from build123d import *
from build123d.topology import SkipClean

# Parameters (mm, degrees)
SKETCH4_R           = 1.524
BOSS_EXTRUDE1_DEPTH = 0.9906
FILLET1_R           = 1.27


with BuildPart() as part:
    # Sketch4 → Boss-Extrude1 (new, symmetric)
    with BuildSketch(Plane.XY):
        with BuildLine():
            Line((-18.252177815, -23.016396438), (-23.016396438, -23.016396438))
            ThreePointArc((-23.016396438, -23.016396438), (-28.612162641, 10.693388458), (0, 29.3751))
            Line((0, 29.3751), (0, 35.7251))
            ThreePointArc((0, 35.7251), (-35.708437486, 1.090991438), (-2.18096518, -35.658465487))
            Line((-2.18096518, -35.658465487), (-1.793306954, -29.320309517))
            ThreePointArc((-1.793306954, -29.320309517), (-10.506673828, -27.431848371), (-18.252177815, -23.016396438))
        make_face()
        with Locations((-7.598669938, -31.650738146)):
            Circle(SKETCH4_R, mode=Mode.SUBTRACT)
    extrude(amount=BOSS_EXTRUDE1_DEPTH, both=True)

    # Fillet1
    fillet1_edges = [part.edges().sort_by_distance(p)[0] for p in [
        (-23.016396438, -23.016396438, 0),
    ]]
    fillet(fillet1_edges, radius=FILLET1_R)

    # Mirror1: part across plane


with BuildPart() as part_1:
    with SkipClean():  # the faces are left unmerged after this step: merging them gives an invalid solid
        add(part.part)
        add(part.part.mirror(Plane(origin=(0, 0, 0), x_dir=(0, 0, 1), z_dir=(1, 0, 0))))


solid = part_1.part
The model under review builds one solid part; all positions refer to its coordinate system, in mm. A direction names the side the tool comes from. Round coordinates to 2 decimals unless told otherwise and drop trailing zeros. Loops run counter-clockwise (first coordinate to the right, second up) from the corner with the lowest first, then second, coordinate; pieces in that order, holes last. Notation, with made-up numbers: M -36.5,3 L -6.5,3 A21 cw -6.5,20 Z; hole C -38,83.5 d6. An arc over 180 degrees is marked long. Answer as CSV lines item,"result". Start each with the question number.
Item 1: For faces 4 (the face through (-5.1, 29.3, 0.991)), 5 (the face through (20, -23.016, 0)), 6 (the face through (-1.99, -32.53, 0.01)), list the 3-axis set-ups (+Z, -Z, +X, -X, +Y, -Y) from which the entire face can be reached by the end or side of a thin tool; tool diameter is ignored.
Item 2: Mouldability with a two-part tool opening along Y and no side actions: class faces 1 (the face through (-5.1, 29.3, -0.991)), 2 (the face through (1.99, -32.53, 0.01)), 3 (the face through (7.8, -30.14, -0.01)) as released by +Y, released by -Y, zero draft, split by the parting line, or undercut.
Item 3: Insertion check: P1, Ø1, axis at x = -19.5, z = 0.5, coming from the +Y side; P2, Ø1, axis at y = 18, z = 0.5, coming from the -X side. Each pin has a flat end and moves straight along its axis. Give the tip position at first contact, or say it passes through.
Item 4: Consider section A-A (y = 0). Write out the cut boundary in (x, z).
Item 5: Consider section B-B (x = 4.5). Write out the cut boundary in (y, z).
Item 6: Consider section C-C (z = 0.4). Write out the cut boundary in (x, y).
Item 7: Wall thickness on line 1 (Y direction, x = 7, z = 0.45); line 2 (Y direction, x = 8, z = -0.2); line 3 (Y direction, x = -18.5, z = -0.8): over which ranges is each line inside the solid? List them lowest first. Write a range as [from, to].
Answer:
1,face 4,"+Z, +X, -X, +Y, -Y"
1,face 5,"+Z, -Z"
1,face 6,"+Z, -Z, -Y"
2,face 1,"zero draft"
2,face 2,"released by -Y"
2,face 3,"undercut"
3,P1,"stops at y = 30.25"
3,P2,"stops at x = -31.15"
4,outline,"M -35.73,-0.99 L -31.2,-0.99 L -31.2,0.99 L -35.73,0.99 Z; M 31.2,-0.99 L 35.73,-0.99 L 35.73,0.99 L 31.2,0.99 Z"
5,outline,"M -35.44,-0.99 L -29.03,-0.99 L -29.03,0.99 L -35.44,0.99 Z; M 29.05,-0.99 L 35.44,-0.99 L 35.44,0.99 L 29.05,0.99 Z"
6,outline,"M -23.4,-22.59 A31.25 cw long 23.4,-22.59 A1.27 cw 22.45,-23.02 L 18.25,-23.02 A29.38 cw 1.79,-29.32 L 2.18,-35.66 A35.73 ccw long -2.18,-35.66 L -1.79,-29.32 A29.38 cw -18.25,-23.02 L -22.45,-23.02 A1.27 cw Z; hole C -7.6,-31.65 d3.05; hole C 7.6,-31.65 d3.05"
7,line 1,"y = [-35.03, -33.05], [-30.25, -28.53], [28.58, 35.03]"
7,line 2,"y = [-34.82, -33.12], [-30.18, -28.26], [28.33, 34.82]"
7,line 3,"y = [-30.56, -23.02], [23.31, 30.56]"
